from build123d import *

# Parameters (mm, degrees)
BOSS_EXTRUDE1_DEPTH = 120
BOSS_EXTRUDE2_DEPTH = 1
SKETCH24_R          = 1.2500000000000002
BOSS_EXTRUDE5_DEPTH = 3
THREAD2_PITCH       = 0.5
SKETCH27_W          = 86
SKETCH27_H          = 6
BOSS_EXTRUDE6_DEPTH = 3
SKETCH28_R          = 1.250000000000001
BOSS_EXTRUDE7_DEPTH = 3
SKETCH29_W          = 46
SKETCH29_H          = 2
SKETCH29_H_2        = 2.000000000000014
SKETCH29_H_3        = 2.0000000000000284
CUT_EXTRUDE1_DEPTH  = 3


with BuildPart() as part:
    # Sketch1 → Boss-Extrude1 (new body)
    with BuildSketch(Plane.XY):
        Polygon((0, 0), (23, 0), (23, 33), (43, 33), (43, 36.00000000000001), (20, 36.00000000000001), (20.000000000000004, 2.9999999999999973), (-19.999999999999996, 2.9999999999999973), (-20, 36.000000000000014), (-43, 36.000000000000014), (-43, 33.00000000000001), (-23, 33), (-23, -2.82e-15), align=None)
    extrude(amount=BOSS_EXTRUDE1_DEPTH)

    # Sketch2 → Boss-Extrude2 (add)
    with BuildSketch(Plane.XY):
        Polygon((-20, 36.000000000000014), (20, 36.000000000000014), (20.000000000000004, 2.9999999999999973), (-19.999999999999996, 2.9999999999999973), align=None)
    extrude(amount=BOSS_EXTRUDE2_DEPTH)

    # Sketch24 → Boss-Extrude5 (add)
    # profile 1 of 2: a face of its own
    with BuildSketch(Plane(origin=(0, 36.000000000000014, 0), x_dir=(1, 0, 0), z_dir=(0, 1, 0))):
        Polygon((-43.000000000000014, 6), (-43, 0), (43, 0), (43, 6.000000000000011), align=None)
        with Locations(Location((0, 3, 0), (0, 0, 270))):
            Circle(SKETCH24_R, mode=Mode.SUBTRACT)
    # profile 2 of 2: a face of its own
    with BuildSketch(Plane(origin=(0, 36.000000000000014, 0), x_dir=(1, 0, 0), z_dir=(0, 1, 0))):
        Polygon((43, 0), (-43, 0), (-43, -120), (-20, -120), (-20, -1), (20, -1.0000000000000009), (20, -120), (43, -120), align=None)
    extrude(amount=-BOSS_EXTRUDE5_DEPTH)

    # Thread2: the profile of 螺纹线轮廓4 profile screwed along a right-hand helix of 6 turns, 6 arcs to a turn; built about Z, then put on its axis
    thread2_z = Axis((0, 0, 0), (0, 0, 1))
    thread2_corners = [(1.2497, 0, -0.000173205), (1.520632938, 0, 0.156249999), (1.520632938, 0, 0.218749999), (1.2497, 0, 0.375173204)]
    with BuildLine(mode=Mode.PRIVATE) as thread2_profile:
        Line(thread2_corners[0], thread2_corners[1])
        Line(thread2_corners[1], thread2_corners[2])
        Line(thread2_corners[2], thread2_corners[3])
        Line(thread2_corners[3], thread2_corners[0])
    thread2_cap = Face(thread2_profile.wire())
    thread2_turn_angles = [0, 30, 60, 90, 120, 150, 180, 210, 240, 270, 300, 330, 360]
    thread2_turn_weights = [1, 0.8660254037844387, 1, 0.8660254037844387, 1, 0.8660254037844387, 1, 0.8660254037844387, 1, 0.8660254037844387, 1, 0.8660254037844387, 1]
    thread2_turn_rails = [Edge.make_bspline([Vector(p[0], p[1], 0).rotate(thread2_z, thread2_turn_angles[k]) / thread2_turn_weights[k] + Vector(0, 0, p[2] + THREAD2_PITCH * thread2_turn_angles[k] / 360) for k in range(13)], [0, 0, 0, 1, 1, 2, 2, 3, 3, 4, 4, 5, 5, 6, 6, 6], 2, thread2_turn_weights) for p in thread2_corners]
    thread2_turn_sides = [Face.make_surface_from_curves(thread2_turn_rails[p[0]], thread2_turn_rails[p[1]]) for p in [(0, 1), (1, 2), (2, 3), (3, 0)]]
    thread2 = Plane(origin=(0, 36, -3), x_dir=(-1, 0, 0), z_dir=(0, -1, 0)) * Solid(Shell([*[p.moved(Location((0, 0, THREAD2_PITCH * i))) for i in range(6) for p in thread2_turn_sides], thread2_cap, thread2_cap.rotate(thread2_z, 2160).moved(Location((0, 0, THREAD2_PITCH * 2160 / 360)))]))
    add(thread2, mode=Mode.SUBTRACT)

    # Sketch27 → Boss-Extrude6 (add)
    with BuildSketch(Plane(origin=(0, 36.000000000000014, 0), x_dir=(1, 0, 0), z_dir=(0, 1, 0))):
        with Locations((-3.55e-15, -123.00000000000001)):
            Rectangle(SKETCH27_W, SKETCH27_H)
    extrude(amount=-BOSS_EXTRUDE6_DEPTH)

    # Sketch28 → Boss-Extrude7 (add)
    with BuildSketch(Plane(origin=(0, 36.000000000000014, 0), x_dir=(1, 0, 0), z_dir=(0, 1, 0))):
        Polygon((-19.999999999999996, -1.0000000000000009), (20.000000000000004, -1.0000000000000009), (20.000000000000004, -37.00000000000001), (-19.99999999999999, -37), align=None)
        with Locations(Location((0, -14.000000000000002, 0), (0, 0, 270))):
            Circle(SKETCH28_R, mode=Mode.SUBTRACT)
    extrude(amount=-BOSS_EXTRUDE7_DEPTH)

    # Sketch29 → Cut-Extrude1 (cut)
    with BuildSketch(Plane(origin=(0, 0, 0), x_dir=(-1, 0, 0), z_dir=(0, -1, 0))):
        Polygon((-23, -5.798088818556618), (23, -5.798088818556618), (23, -20.798088818556618), (-22.999999999999996, -20.798088818556618), align=None)
        with Locations((0, -44.19328812281581)):
            Rectangle(SKETCH29_W, SKETCH29_H)
        with Locations((1.0303e-13, -54.193288122815815)):
            Rectangle(SKETCH29_W, SKETCH29_H_2)
        with Locations((3.1264e-13, -74.19328812281582)):
            Rectangle(SKETCH29_W, SKETCH29_H)
        with Locations((4.1567e-13, -84.19328812281582)):
            Rectangle(SKETCH29_W, SKETCH29_H)
        with Locations((6.2528e-13, -104.19328812281582)):
            Rectangle(SKETCH29_W, SKETCH29_H_3)
        with Locations((7.2831e-13, -114.19328812281583)):
            Rectangle(SKETCH29_W, SKETCH29_H)
    extrude(amount=-CUT_EXTRUDE1_DEPTH, mode=Mode.SUBTRACT)


solid = part.part
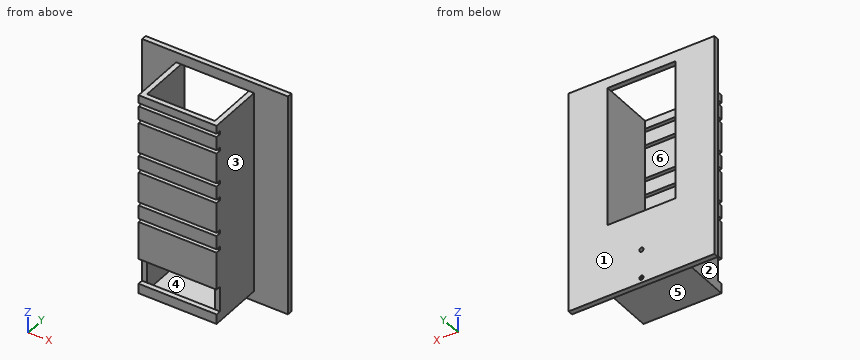
Geometry: final body of the model. Coordinates: model frame, mm. Face numbers are marked on the shaded views. A direction names the side the tool comes from. Give positions to 0.01 mm unless a question says otherwise; leave off trailing zeros. Write each loop counter-clockwise with the first axis right and the second up, starting at its lowest first coordinate (ties: lowest second). Pieces come first, ordered by that corner, then holes. Notation, with made-up numbers: M 13,18.25 L 37,18.25 A23 ccw 37,56.25 Z; hole C 33,-24.75 d10. An arc over 180 degrees is marked long. Answer in a Markdown table with one row per item. Add a question column.
(1) Reachability of the marked faces 1, 2 and 3 from +Z, -Z, +X, -X, +Y, -Y: full face, straight path, thin tool, end or side. Return the list, or none.
(2) Section A-A on z = 28. Return loops of the section in (x, y), and give its area (3 significant figures).
(3) Mould query, pull axis Y, two halves, no side actions, for the marked faces 4, 5 and 6. Classes: +Y half, -Y half, draft (parallel to the pull), parting line (faces both ways), or undercut.
(4) Section D-D on x = -30.5. Return loops of the section in (y, z).
(5) Section B-B on z = 117. Return loops of the section in (x, y), and give its area (3 significant figures).
(6) First-contact query: pin 1 (16.5 mm diameter, centred on x = -11, y = 24.5, fed in from -Z); pin 2 (3 mm diameter, centred on y = 27.5, z = 50.5, fed in from -X); pin 3 (1.5 mm diameter, centred on x = 21, z = 17, fed in from -Y). Flat tips, straight axial feed; report the tip coordinate or a pass-through.
(7) Section C-C on y = 26. Return loops of the section in (x, z), and give its area (3 significant figures).
(8) Ray query, line 1 (X direction, y = 7, z = 92); line 2 (X direction, y = 35.35, z = -3); line 3 (Y direction, x = 36.5, z = 89). Return the intervals inside material, ascending.
Result set:
| question | item | result |
|---|---|---|
| 1 | face 1 | +Z, -Z, +X, -X, +Y |
| 1 | face 2 | +Z, -Z, -X, -Y |
| 1 | face 3 | +Z, -Z, +X, -Y |
| 2 | outline | M -43,33 L -23,33 L -23,0 L 23,0 L 23,33 L 43,33 L 43,36 L -43,36 Z; hole M -20,3 L 20,3 L 20,33 L -20,33 Z |
| 2 | area | 576 mm^2 |
| 3 | face 4 | undercut |
| 3 | face 5 | draft |
| 3 | face 6 | +Y half |
| 4 | outline | M 33,-6 L 36,-6 L 36,126 L 33,126 Z |
| 5 | outline | M -43,33 L -23,33 L -23,0 L 23,0 L 23,33 L 43,33 L 43,36 L 20,36 L 20,3 L -20,3 L -20,36 L -43,36 Z |
| 5 | area | 456 mm^2 |
| 6 | pin 1 | stops at z = 0 |
| 6 | pin 2 | stops at x = -23 |
| 6 | pin 3 | stops at y = 3 |
| 7 | outline | M -23,0 L 23,0 L 23,120 L 20,120 L 20,1 L -20,1 L -20,120 L -23,120 Z |
| 7 | area | 760 mm^2 |
| 8 | line 1 | x = -23 to -20, 20 to 23 |
| 8 | line 2 | x = -43 to -1.51, 1.25 to 43 |
| 8 | line 3 | y = 33 to 36 |
